from build123d import *

# Parameters (mm, degrees)
BOSS_EXTRUDE1_DEPTH = 10
SKETCH2_R           = 1.5
CUT_EXTRUDE1_DEPTH  = 13
CUT_EXTRUDE2_START  = -13
SKETCH3_R           = 1.5
CUT_EXTRUDE2_DEPTH  = 13
SKETCH4_R           = 2.5
BOSS_EXTRUDE2_DEPTH = 10
SKETCH5_R           = 3.5
BOSS_EXTRUDE3_DEPTH = 5
SKETCH6_R           = 1.25
CUT_EXTRUDE3_DEPTH  = 4


with BuildPart() as part:
    # Sketch1 → Boss-Extrude1 (new body)
    with BuildSketch(Plane.XY):
        Polygon((-14.5, 2.6), (-7.7, 2.6), (-7.7, 5), (-6.767766953, 5), (-4.4, 2.632233047), (-4.4, -2.632233047), (-6.767766953, -5), (-7.7, -5), (-7.7, -2.6), (-10.5, -2.6), (-10.5, -10.5), (30.5, -10.5), (30.5, -2.6), (27.7, -2.6), (27.7, -5), (26.767766953, -5), (24.4, -2.632233047), (24.4, 2.632233047), (26.767766953, 5), (27.7, 5), (27.7, 2.6), (34.5, 2.6), (34.5, -14.5), (15, -14.5), (15, -55), (5, -55), (5, -14.5), (-14.5, -14.5), align=None)
    extrude(amount=BOSS_EXTRUDE1_DEPTH)

    # Sketch2 → Cut-Extrude1 (cut)
    with BuildSketch(Plane.ZY.offset(14.5)):
        with Locations(Location((5, 0, 0), (0, 0, 270))):
            Circle(SKETCH2_R)
    extrude(amount=-CUT_EXTRUDE1_DEPTH, mode=Mode.SUBTRACT)

    # Sketch3 → Cut-Extrude2 (cut)
    with BuildSketch(Plane(origin=(34.5, 0, 0), x_dir=(0, 0, -1), z_dir=(1, 0, 0)).offset(CUT_EXTRUDE2_START)):
        with Locations(Location((-5, 0, 0), (0, 0, 270))):
            Circle(SKETCH3_R)
    extrude(amount=CUT_EXTRUDE2_DEPTH, mode=Mode.SUBTRACT)

    # Sketch4 → Boss-Extrude2 (add)
    with BuildSketch(Plane.XY.offset(10)):
        with Locations((10, -49)):
            Circle(SKETCH4_R)
    extrude(amount=BOSS_EXTRUDE2_DEPTH)

    # Sketch5 → Boss-Extrude3 (add)
    with BuildSketch(Plane.XY.offset(10)):
        with Locations((10, -49)):
            Circle(SKETCH5_R)
    extrude(amount=BOSS_EXTRUDE3_DEPTH)

    # Sketch6 → Cut-Extrude3 (cut)
    with BuildSketch(Plane.XY.offset(20)):
        with Locations((10, -49)):
            Circle(SKETCH6_R)
    extrude(amount=-CUT_EXTRUDE3_DEPTH, mode=Mode.SUBTRACT)


solid = part.part
Geometry check sheet. Reference: the model listing, model coordinates, mm. A direction names the side the tool comes from. Round coordinates to 2 decimals unless told otherwise and drop trailing zeros. Write each loop counter-clockwise with the first axis right and the second up, starting at its lowest first coordinate (ties: lowest second). Pieces come first, ordered by that corner, then holes. Notation, with made-up numbers: (20, 35) - (61, 35) arc R25 cw to (61, 48) - close; hole circle Ø2 at (20.5, 56). An arc over 180 degrees is marked (long way). One line per item, written item: value.
1. Depth check by flat-ended pin: pin 1 Ø3 at (x, z) = (18, 3) entering from +Y; pin 2 Ø10 at (x, y) = (12.5, -36.5) entering from +Z; pin 3 Ø12 at (x, y) = (-2.5, -42) entering from +Z; pin 4 Ø3 at (y, z) = (-29.5, 5) entering from -X. Enter the tip coordinate at first touch or a pass-through.
The answers:
pin 1: stops at y = -10.5
pin 2: stops at z = 10
pin 3: passes through
pin 4: stops at x = 5
2. Cross-section at A-A on y = 0. Record the boundary of the cut face in (x, z), and give its area (3 significant figures).
The answers:
outline: (-14.5, 0) - (-4.4, 0) - (-4.4, 3.5) - (-14.5, 3.5) - close; (-14.5, 6.5) - (-4.4, 6.5) - (-4.4, 10) - (-14.5, 10) - close; (24.4, 0) - (34.5, 0) - (34.5, 3.5) - (24.4, 3.5) - close; (24.4, 6.5) - (34.5, 6.5) - (34.5, 10) - (24.4, 10) - close
area: 141 mm^2
3. Cross-section at B-B on x = 28.5. Record the boundary of the cut face in (y, z), and give its area (3 significant figures).
The answers:
outline: (-14.5, 0) - (-10.5, 0) - (-10.5, 10) - (-14.5, 10) - close; (-2.6, 0) - (2.6, 0) - (2.6, 10) - (-2.6, 10) - close; hole circle Ø3 at (0, 5)
area: 84.9 mm^2
4. Cross-section at D-D on x = 10. Record the boundary of the cut face in (y, z), and give its area (3 significant figures).
The answers:
outline: (-55, 0) - (-10.5, 0) - (-10.5, 10) - (-45.5, 10) - (-45.5, 15) - (-46.5, 15) - (-46.5, 20) - (-47.75, 20) - (-47.75, 16) - (-50.25, 16) - (-50.25, 20) - (-51.5, 20) - (-51.5, 15) - (-52.5, 15) - (-52.5, 10) - (-55, 10) - close
area: 495 mm^2
5. Mould release check, pull along X, two halves, no side actions. Record for faces 6 (the face through (-4.4, 1.2, 3.8)), 7 (the face through (9.46, -51.44, 17.46)), 8 (the face through (-11, 2.6, 5)), 9 (the face through (-14.5, -6, 5)): released by +X, released by -X, zero draft, split by the parting line, or undercut.
The answers:
face 6: undercut
face 7: split by the parting line
face 8: zero draft
face 9: released by -X
6. Scan lines: L1, parallel to Y at x = 27.5, z = 5; L2, parallel to Y at x = 29, z = 5; L3, parallel to Y at x = 10, z = 18.6. Record each from-to range of solid material in increasing order.
The answers:
L1: y = -14.5 to -10.5, -5 to -1.5, 1.5 to 5
L2: y = -14.5 to -10.5, -2.6 to -1.5, 1.5 to 2.6
L3: y = -51.5 to -50.25, -47.75 to -46.5
7. Cross-section at C-C on z = 7.75. Record the boundary of the cut face in (x, y), and give its area (3 significant figures).
The answers:
outline: (-14.5, -14.5) - (5, -14.5) - (5, -55) - (15, -55) - (15, -14.5) - (34.5, -14.5) - (34.5, 2.6) - (27.7, 2.6) - (27.7, 5) - (26.77, 5) - (24.4, 2.63) - (24.4, -2.63) - (26.77, -5) - (27.7, -5) - (27.7, -2.6) - (30.5, -2.6) - (30.5, -10.5) - (-10.5, -10.5) - (-10.5, -2.6) - (-7.7, -2.6) - (-7.7, -5) - (-6.77, -5) - (-4.4, -2.63) - (-4.4, 2.63) - (-6.77, 5) - (-7.7, 5) - (-7.7, 2.6) - (-14.5, 2.6) - close
area: 790 mm^2
8. Set-up check for faces 1 (the face through (-7.7, -4, 5)), 2 (the face through (-7.7, 4, 5)), 3 (the face through (9.84, -47.76, 18.03)), 4 (the face through (25.57, 3.8, 4.93)), 5 (the face through (5, -35, 5)): record each of +Z, -Z, +X, -X, +Y, -Y from which the full face is reachable in a straight line by a thin tool's end or side.
The answers:
face 1: +Z, -Z
face 2: +Z, -Z, -X, +Y
face 3: +Z
face 4: +Z, -Z, +Y
face 5: +Z, -Z, -X, -Y
